Here's how the part is built. I have some questions about the finished solid (model axes, mm). A direction names the side the tool comes from. Coordinates: 2 decimals unless noted, no trailing zeros. Write each loop counter-clockwise with the first axis right and the second up, starting at its lowest first coordinate (ties: lowest second). Pieces come first, ordered by that corner, then holes.
Item 1: I want a section at C-C (y = 70). Please give me the cut outline in (x, z).
Item 2: I'm going to push flat-ended pins straight in: P1, Ø4, axis at x = -29.5, y = -20.5, coming from the +Z side; P2, Ø0.8, axis at x = -18.5, z = -1.5, coming from the -Y side; P3, Ø11, axis at y = 155.5, z = 11, coming from the -X side. Where does each tip first touch, or does it pass through?
Item 3: I want a section at A-A (x = -16). Please give me the cut outline in (y, z), and give its area (3 significant figures).
Item 4: I want a section at B-B (y = 155). Please give me the cut outline in (x, z).
Item 5: If we mould it in two halves opening along X, with no side actions, what happens to faces 3 (the face through (0, -78, 18)), 4 (the face through (-17.201, -151.185, -1.972)), 5 (the face through (4, 2, -1))? For each: pulls with the +X half, pulls with the -X half, needs draft (parallel to the pull), parting line crosses it, or undercut.
Item 6: For faces 1 (the face through (-14.799, 151.185, -1.972)), 2 (the face through (0, 80, 18)), which set-ups out of +Z, -Z, +X, -X, +Y, -Y let a thin tool reach every point of the face, with its end or its side?
Item 7: Please list where these lines run through material, in increasing order: line 1 (Z direction, x = 2.7, y = -39); line 2 (X direction, y = 155, z = -2); line 3 (Z direction, x = -32.5, y = 26).
Solid Edge part; units mm, degrees
sketch "Sketch1" plane through (0, 0, 0) normal (0, -1, 0) x (1, 0, 0)
  line L0 (-36, 0) -> (0, 0)
  line L1 (0, 0) -> (0, 36)
  line L2 (0, 36) -> (4, 36)
  line L3 (4, 36) -> (4, -4)
  line L4 (4, -4) -> (-36, -4)
  line L5 (-36, -4) -> (-36, 0)
extrude "Protrusion1" add sketch "Sketch1" along normal mid plane 350
sketch "Sketch2" plane through (-18, 0, 0) normal (0, 0, 1) x (0, -1, 0)
  circle A0 centre (-155, 2) radius 4
  dimension "D1" = 155
  dimension "D2" = 155
extrude "Cutout1" cut sketch "Sketch2" against normal through all
mirror "Mirror1" about plane through (0, 0, 0) normal (0, -1, 0) of "Cutout1"
sketch "Sketch3" plane through (0, 0, 18) normal (-1, 0, 0) x (0, -1, 0)
  line L0 (-22.5, -18) -> (22.5, -18)
  line L1 (22.5, -18) -> (22.5, 18)
  line L2 (22.5, 18) -> (-22.5, 18)
  line L3 (-22.5, 18) -> (-22.5, -18)
  dimension "D1" = 22.5
extrude "Cutout2" cut sketch "Sketch3" against normal through all
sketch "Sketch4" plane through (0, -97.75, 18) normal (-1, 0, 0) x (0, -1, 0)
  circle A0 centre (-58.75, 5) radius 2.5
  circle A1 centre (-58.75, -10) radius 2.5
  dimension "D1" = 58.75
extrude "Cutout3" cut sketch "Sketch4" against normal through all
sketch "Sketch5" plane through (-16, 0, 0) normal (0, 0, 1) x (0, 1, 0)
  line L0 (175, 20) -> (171, 20)
  line L1 (171, 20) -> (171, -16)
  line L2 (171, -16) -> (175, -16)
  line L3 (175, -16) -> (175, 20)
  dimension "D1" = 175
extrude "Cutout4" cut sketch "Sketch5" against normal up to next
sketch "Sketch6" plane through (4, 0, 16) normal (1, 0, 0) x (0, 1, 0)
  line L0 (139, 20) -> (135, 20)
  line L1 (135, 20) -> (135, -16)
  line L2 (135, -16) -> (139, -16)
  line L3 (139, -16) -> (139, 20)
  dimension "D1" = 139
extrude "Cutout5" cut sketch "Sketch6" against normal up to next
sketch "Sketch7" plane through (-16, -2, 0) normal (0, 0, 1) x (0, 1, 0)
  line L0 (-173, 20) -> (-169, 20)
  line L1 (-169, 20) -> (-169, -16)
  line L2 (-169, -16) -> (-173, -16)
  line L3 (-173, -16) -> (-173, 20)
  dimension "D1" = 173
extrude "Cutout6" cut sketch "Sketch7" against normal up to next
sketch "Sketch8" plane through (4, 0, 16) normal (1, 0, 0) x (0, 1, 0)
  line L0 (-139, 20) -> (-135, 20)
  line L1 (-135, 20) -> (-135, -16)
  line L2 (-135, -16) -> (-139, -16)
  line L3 (-139, -16) -> (-139, 20)
  dimension "D1" = 139
extrude "Cutout7" cut sketch "Sketch8" against normal up to next
chamfer "Fase_3" distance 1.5 angle 45 4 edges at (4, 139, 18) (4, -139, 18) (-18, 171, -4) (-18, -171, -4)
properties material "Aluminium, 7075-T6"
Answer:
1. outline: (-36, -4) - (4, -4) - (4, 36) - (0, 36) - (0, 0) - (-36, 0) - close
2. P1: stops at z = 0
2. P2: stops at y = -171
2. P3: stops at x = 0
3. outline: (-171, -2.5) - (-169.5, -4) - (-159, -4) - (-159, 0) - (-171, 0) - close; (-151, -4) - (151, -4) - (151, 0) - (-151, 0) - close; (159, -4) - (169.5, -4) - (171, -2.5) - (171, 0) - (159, 0) - close
3. area: 1,300 mm2
4. outline: (-36, -4) - (-20, -4) - (-20, 0) - (-36, 0) - close; (-12, -4) - (4, -4) - (4, 36) - (0, 36) - (0, 0) - (-12, 0) - close
5. face 3: pulls with the -X half
5. face 4: undercut
5. face 5: pulls with the +X half
6. face 1: +Z, -Z
6. face 2: +Z, -X, +Y, -Y
7. line 1: z = -4 to 5.5, 10.5 to 20.5, 25.5 to 36
7. line 2: x = -36 to -20, -12 to 4
7. line 3: z = -4 to 0
